Read the model definition and answer for the solid it produces. Units are mm, in the model's axes. Round coordinates to 2 decimals unless told otherwise and drop trailing zeros.
from build123d import *

# Parameters (mm, degrees)
SKETCH1_W           = 250
SKETCH1_H           = 55
BOSS_EXTRUDE1_DEPTH = 3.175


with BuildPart() as part:
    # Sketch1 → Boss-Extrude1 (new body)
    with BuildSketch(Plane.XY):
        with Locations((-241.58829827, -18.367364772)):
            Rectangle(SKETCH1_W, SKETCH1_H)
        with BuildLine():
            Line((-278.807431502, -11.635308713), (-260.807431502, -11.635308713))
            Line((-260.807431502, -11.635308713), (-260.807431502, -25.094140403))
            Line((-260.807431502, -25.094140403), (-278.708074604, -25.094140403))
            add(Edge.make_bspline(
                [(-278.807431502, -11.635308713), (-278.842567637, -11.635308713), (-278.877724877, -11.635597737), (-279.131916675, -11.639782512), (-279.34983121, -11.654506754), (-279.783435066, -11.706373741), (-280.000022761, -11.743764607), (-280.637043124, -11.888179154), (-281.046210232, -12.026893167), (-281.834248732, -12.387198003), (-282.214784616, -12.611112168), (-282.91286176, -13.122553874), (-283.23487643, -13.411547156), (-283.824414261, -14.056624874), (-284.084709523, -14.405325127), (-284.420910809, -14.959373126), (-284.524173104, -15.149599512), (-284.712815972, -15.541311056), (-284.798455074, -15.743725981), (-285.023266518, -16.356140938), (-285.132324707, -16.77404955), (-285.270965185, -17.628621863), (-285.299780117, -18.068728441), (-285.276335696, -18.934229846), (-285.225127225, -19.363108441), (-285.086887053, -20.000402626), (-285.030151101, -20.212732347), (-284.897978299, -20.627014671), (-284.822460465, -20.829775079), (-284.568196741, -21.425185334), (-284.362007249, -21.805088054), (-283.873373823, -22.529474489), (-283.596617119, -22.864951248), (-283.139203055, -23.322938066), (-282.979382751, -23.468376569), (-282.6446555, -23.744423912), (-282.468681353, -23.875710362), (-281.925950724, -24.240109672), (-281.545469248, -24.444161396), (-280.747183384, -24.774500883), (-280.324174276, -24.901275116), (-279.505292308, -25.056948004), (-279.108516523, -25.094140403), (-278.708074604, -25.094140403)],
                knots=[0.997490672, 0.997490672, 0.997490672, 0.997490672, 1, 1, 1.015625, 1.015625, 1.03125, 1.03125, 1.0625, 1.0625, 1.09375, 1.09375, 1.125, 1.125, 1.15625, 1.15625, 1.171875, 1.171875, 1.1875, 1.1875, 1.21875, 1.21875, 1.25, 1.25, 1.28125, 1.28125, 1.296875, 1.296875, 1.3125, 1.3125, 1.34375, 1.34375, 1.375, 1.375, 1.390625, 1.390625, 1.40625, 1.40625, 1.4375, 1.4375, 1.46875, 1.46875, 1.497597951, 1.497597951, 1.497597951, 1.497597951], degree=3))
        make_face(mode=Mode.SUBTRACT)
        with BuildLine():
            Line((-154.360316654, -11.635298321), (-136.360316654, -11.635298321))
            Line((-136.360316654, -11.635298321), (-136.360316654, -25.09414087))
            Line((-136.360316654, -25.09414087), (-154.458489548, -25.09414087))
            add(Edge.make_bspline(
                [(-154.360316654, -11.635298321), (-154.761727997, -11.635298321), (-155.157386504, -11.672727127), (-155.759665345, -11.787140661), (-155.970243269, -11.838376709), (-156.387966493, -11.963181969), (-156.594872022, -12.036850346), (-157.196347851, -12.28608082), (-157.576755859, -12.490915834), (-158.117253538, -12.854781423), (-158.293226627, -12.986353957), (-158.628820603, -13.263982392), (-158.788816486, -13.410133743), (-159.246155666, -13.869889244), (-159.521251185, -14.204841131), (-160.009167015, -14.931608928), (-160.214692704, -15.312488329), (-160.467795081, -15.908929825), (-160.542897196, -16.111961519), (-160.674225623, -16.52661774), (-160.730530769, -16.739037016), (-160.867597895, -17.37656092), (-160.918148194, -17.805473824), (-160.940601815, -18.670806399), (-160.911402505, -19.110937169), (-160.772322277, -19.965020543), (-160.663242958, -20.382313943), (-160.438953589, -20.993295919), (-160.353444122, -21.195550415), (-160.164485449, -21.587994273), (-160.061148171, -21.778323473), (-159.725133032, -22.332012421), (-159.46672666, -22.678256324), (-158.877844125, -23.322799834), (-158.553373423, -23.613738751), (-158.031112315, -23.995810431), (-157.850620858, -24.114523058), (-157.476451569, -24.334149523), (-157.281538298, -24.435580841), (-156.686819382, -24.706814458), (-156.277513308, -24.844436489), (-155.433635452, -25.034586177), (-154.994831316, -25.08641844), (-154.527357053, -25.093865983), (-154.492916253, -25.09414087), (-154.458489548, -25.09414087)],
                knots=[0.002538772, 0.002538772, 0.002538772, 0.002538772, 0.03125, 0.03125, 0.046875, 0.046875, 0.0625, 0.0625, 0.09375, 0.09375, 0.109375, 0.109375, 0.125, 0.125, 0.15625, 0.15625, 0.1875, 0.1875, 0.203125, 0.203125, 0.21875, 0.21875, 0.25, 0.25, 0.28125, 0.28125, 0.3125, 0.3125, 0.328125, 0.328125, 0.34375, 0.34375, 0.375, 0.375, 0.40625, 0.40625, 0.421875, 0.421875, 0.4375, 0.4375, 0.46875, 0.46875, 0.5, 0.5, 0.502486526, 0.502486526, 0.502486526, 0.502486526], degree=3))
        make_face(mode=Mode.SUBTRACT)
    extrude(amount=BOSS_EXTRUDE1_DEPTH)


solid = part.part
Q1. Flat-ended cylindrical pins translate along their axes: pin 1 (10 mm diameter, centred on x = -307, y = -26, fed in from -Z); pin 2 (8 mm diameter, centred on x = -156, y = -20, fed in from -Z). Find the tip coordinate at first contact, or state that the pin passes through.
Outcome:
pin 1: stops at z = 0
pin 2: passes through
Q2. Straight lines are drawn through the part: probe 1 along X at (y, z) = (-19.5, 1.85); probe 2 along Y at (x, z) = (-151.5, 1.05); probe 3 along X at (y, z) = (-17.5, 3). For each, find the intervals that lie inside material, in ascending order.
Outcome:
probe 1: x = -366.59 to -285.19, -260.81 to -160.85, -136.36 to -116.59
probe 2: y = -45.87 to -25.09, -11.64 to 9.13
probe 3: x = -366.59 to -285.24, -260.81 to -160.87, -136.36 to -116.59
Q3. A cutting plane is placed at A-A, the plane z = 2.55. Give the number of separate pieces and of enclosed holes in the cut face, plus the area to 3 significant figures.
Outcome:
separate pieces: 1
enclosed holes: 2
area: 13,100 mm2
